The drawing under review shows one solid part. Ordinate dimensions are in mm from its lowest x, y, z. A direction names the side the tool comes from. Coordinates: 2 decimals unless noted, no trailing zeros. Loops run counter-clockwise (first coordinate to the right, second up) from the corner with the lowest first, then second, coordinate; pieces in that order, holes last.
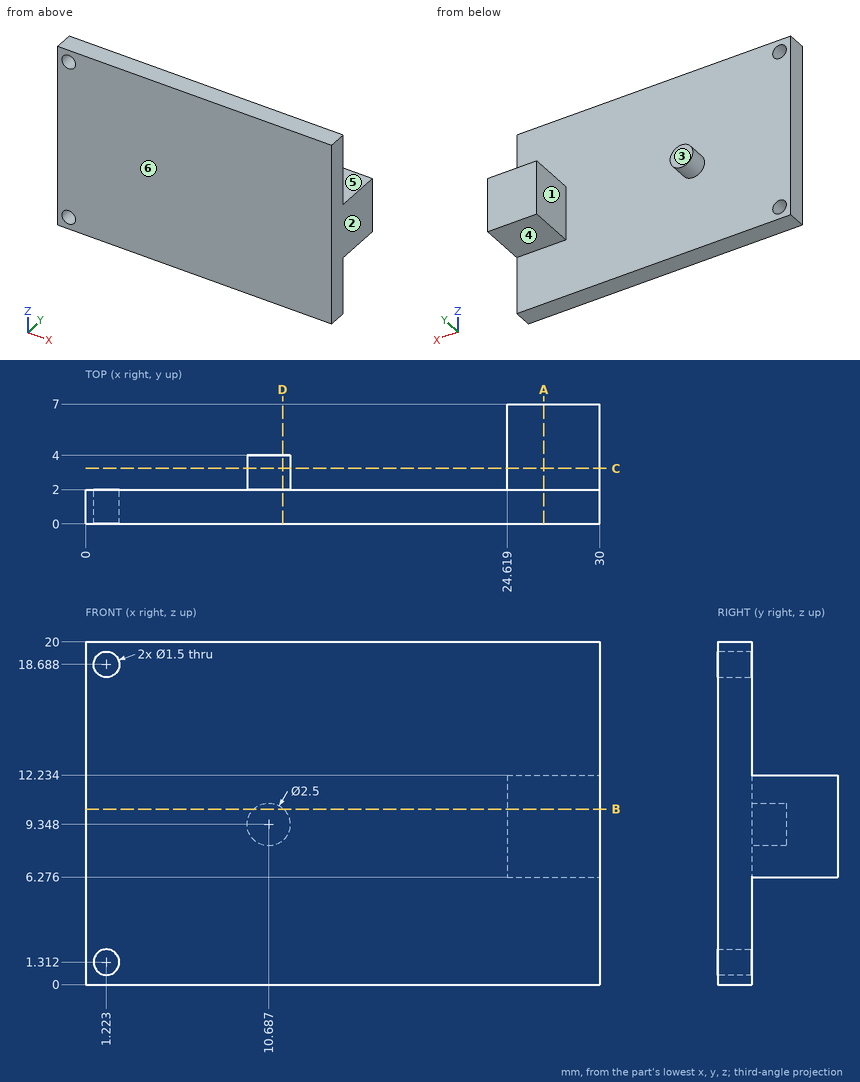
Q1. For line 1 (Y direction, x = 12.5, z = 6); line 2 (X direction, y = 5, z = 9.75); line 3 (X direction, y = 1.25, z = 1.5), list the stretches that pass through material, from the lowest coordinate up.
Q2. Take a section at C-C, the plane y = 3.25. Write out the cut boundary in (x, z).
Q3. Machinability: for the marked faces 4, 5 and 6, which of the approach directions +Z, -Z, +X, -X, +Y, -Y give a long, thin tool a straight path to every point of the face, cutting with its end or side? Answer none if there is none.
Q4. Take a section at A-A, the plane x = 26.75. Write out the cut boundary in (y, z).
Q5. Take a section at D-D, the plane x = 11.5. Write out the cut boundary in (y, z), then the cut area to 3 significant figures.
Q6. Clearance check with flat-ended pins moving along their axes: pin 1 Ø3 at (x, y) = (9, 4) entering from -Z; pin 2 Ø4 at (y, z) = (5.5, 9) entering from -X; pin 3 Ø2 at (x, y) = (9, 3.5) entering from +Z. State where each tip first meets the part, or that it passes through.
Q7. The part is to be moulded in two halves that separate along X. For the marked faces 1, 2 and 3, say which applies: pulls with the +X half, pulls with the -X half, needs draft (parallel to the pull), parting line crosses it, or undercut.
Q8. Take a section at B-B, the plane z = 10.25. Write out the cut boundary in (x, y).
Entries:
1. line 1: y = 0 to 2
1. line 2: x = 24.62 to 30
1. line 3: x = 0 to 0.5, 1.95 to 30
2. outline: circle Ø2.5 at (10.69, 9.35); (24.62, 6.28) - (30, 6.28) - (30, 12.23) - (24.62, 12.23) - close
3. face 4: -Z, +X, -X, +Y
3. face 5: +Z, +X, -X, +Y
3. face 6: +Z, -Z, +X, -X, -Y
4. outline: (0, 0) - (2, 0) - (2, 6.28) - (7, 6.28) - (7, 12.23) - (2, 12.23) - (2, 20) - (0, 20) - close
5. outline: (0, 0) - (2, 0) - (2, 8.4) - (4, 8.4) - (4, 10.3) - (2, 10.3) - (2, 20) - (0, 20) - close
5. area: 43.8 mm2
6. pin 1: stops at z = 8.11
6. pin 2: stops at x = 9.44
6. pin 3: stops at z = 10.39
7. face 1: undercut
7. face 2: pulls with the +X half
7. face 3: needs draft
8. outline: (0, 0) - (30, 0) - (30, 7) - (24.62, 7) - (24.62, 2) - (11.55, 2) - (11.55, 4) - (9.82, 4) - (9.82, 2) - (0, 2) - close
